Input: dimensioned drawing with shaded views. Units: mm. Origin: part minimum x, y, z. Coordinates: 2 decimals unless noted, no trailing zeros. Loops run counter-clockwise (first coordinate to the right, second up) from the corner with the lowest first, then second, coordinate; pieces in that order, holes last.
Item 1: Section D-D on z = 19. Return loops of the section in (x, y) (1 decimal).
Item 2: Section A-A on y = 17. Return loops of the section in (x, z) (1 decimal).
Item 3: Ray query, line 1 along Z through (x, y) = (2.2, 21.25) (1 decimal); line 2 along Z through (x, y) = (1.95, 14.75) (1 decimal); line 3 along Y through (x, z) = (0.7, 42) (1 decimal). Return the intervals inside material, ascending.
Item 4: Section B-B on x = 2.2. Give the number of separate pieces and of enclosed holes in the cut face.
Item 5: Section C-C on z = 12. Return loops of the section in (x, y) (1 decimal).
Item 6: Contact query for a flat-ended pin moving along its axis: P1, Ø1.6, axis at x = 2.5, y = 18, coming from the -Z side (1 decimal). Output: stop coordinate, or through.
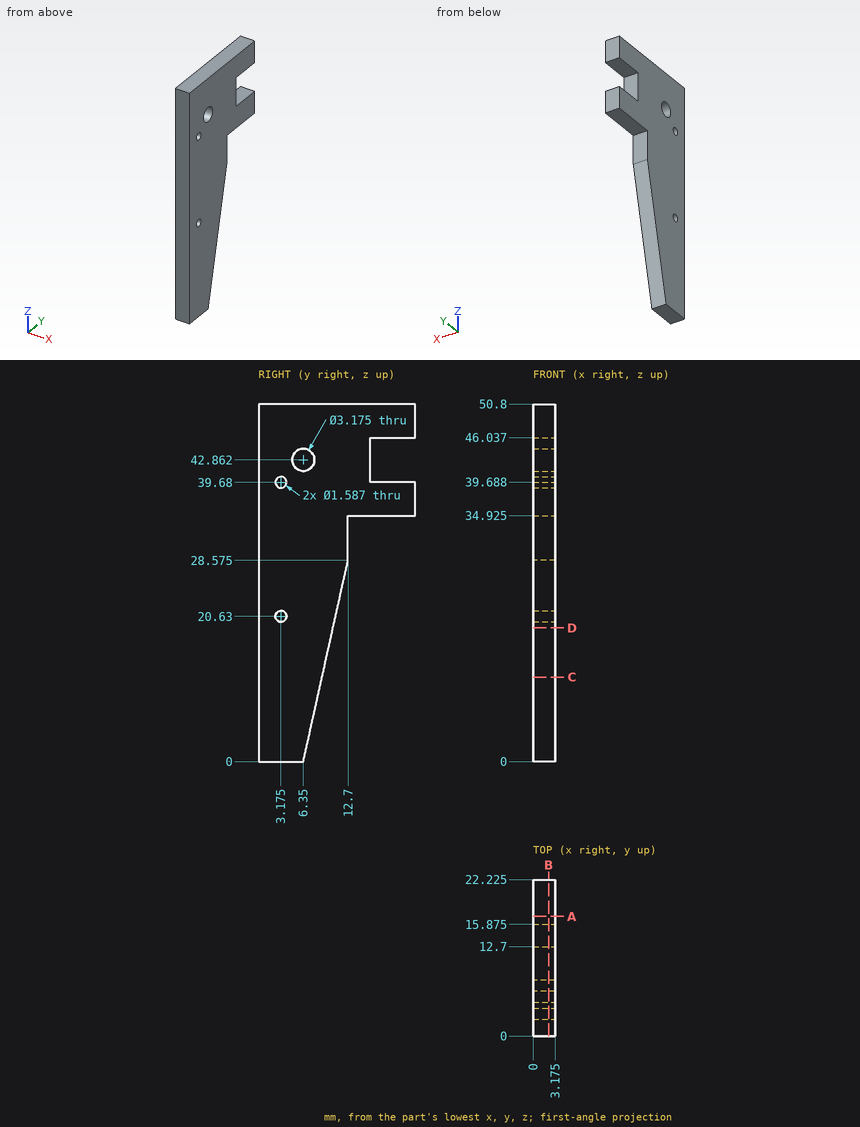
Results found:
1. outline: (0, 0) - (3.2, 0) - (3.2, 10.6) - (0, 10.6) - close
2. outline: (0, 34.9) - (3.2, 34.9) - (3.2, 39.7) - (0, 39.7) - close; (0, 46) - (3.2, 46) - (3.2, 50.8) - (0, 50.8) - close
3. line 1: z = 34.9 to 39.7, 46 to 50.8
3. line 2: z = 34.9 to 50.8
3. line 3: y = 0 to 5, 7.7 to 15.9
4. separate pieces: 1
4. enclosed holes: 3
5. outline: (0, 0) - (3.2, 0) - (3.2, 9) - (0, 9) - close
6. P1: stops at z = 34.9
